Geometry: see drawing. Coordinates: mm, zero at the bounding-box minimum. A direction names the side the tool comes from. Coordinates: 2 decimals unless noted, no trailing zeros. Loops run counter-clockwise (first coordinate to the right, second up) from the corner with the lowest first, then second, coordinate; pieces in that order, holes last. Notation, with made-up numbers: (-19.5, 0.5) -> (3.5, 0.5) arc R22 cw to (3.5, 14.5) -> close; hole circle Ø1 at (-32, 85.5). An arc over 180 degrees is marked (long way). One line per item, written item: value. Start each with the question number.
Item 1: Ray query, probe 1 along Y at (x, z) = (12.7, 4.25); probe 2 along Z at (x, y) = (44.5, 12.7) (3 decimals); probe 3 along Z at (x, y) = (5, 9.5). Return the intervals inside material, ascending. Write a range as from..to.
Item 2: Mould query, pull axis X, two halves, no side actions, for the marked faces 4, 5 and 6. Classes: +X half, -X half, draft (parallel to the pull), parting line (faces both ways), or undercut.
Item 3: Section query D-D on x = 17. Return loops of the section in (y, z).
Item 4: Contact query for flat-ended pins moving along their axis: pin 1 Ø10 at (y, z) = (4.5, 36.5) entering from +X; pin 2 Ø1 at (y, z) = (20, 7.5) entering from -X; pin 3 Ø3 at (y, z) = (7.5, 13) entering from -X; pin 4 Ø11.5 at (y, z) = (12.7, 28.575) entering from -X. Output: stop coordinate, or through.
Item 5: Set-up query: the marked faces 1, 2 and 3. Return all of +Z, -Z, +X, -X, +Y, -Y with unobstructed straight access to the full face (end or side cutting, diameter ignored); none if empty.
Item 6: Section query A-A on y = 17.5. Return loops of the section in (x, z).
Item 7: Section query B-B on z = 32. Return loops of the section in (x, y).
Item 8: Section query C-C on x = 47. Return loops of the section in (y, z) (3 decimals).
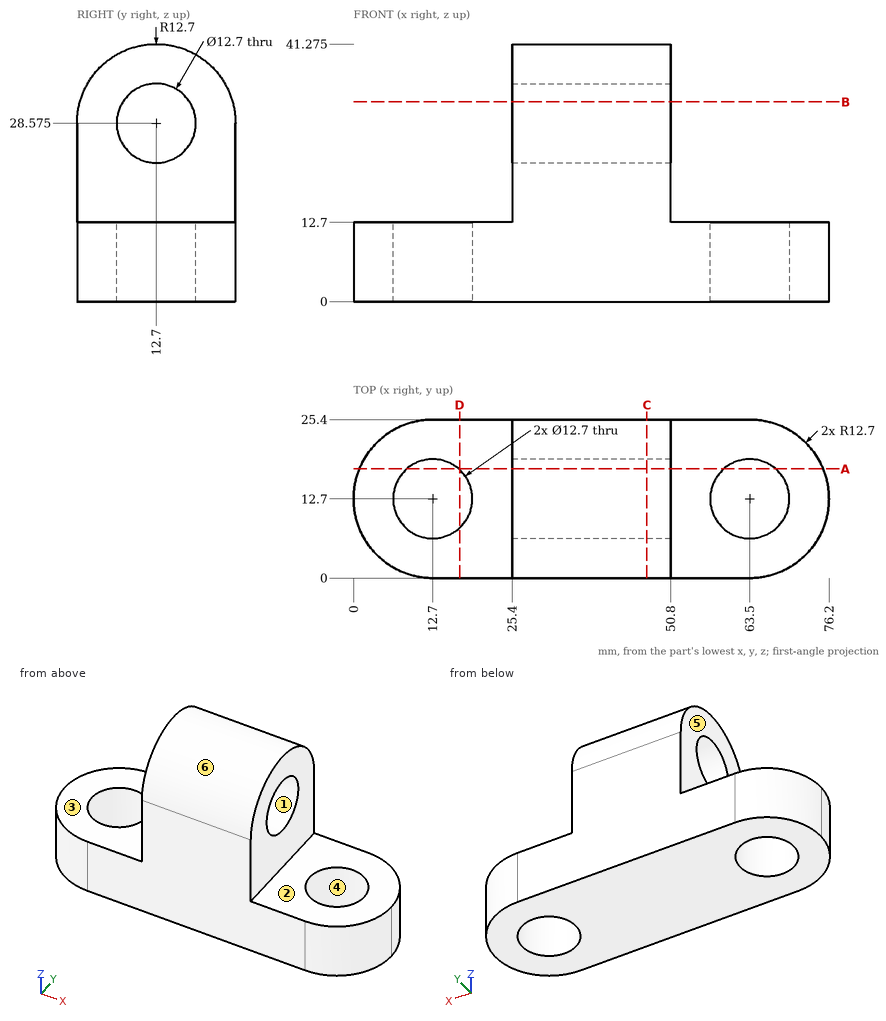
Reply:
1. probe 1: y = 0..6.35, 19.05..25.4
1. probe 2: z = 0..22.225, 34.925..41.275
1. probe 3: z = 0..12.7
2. face 4: undercut
2. face 5: -X half
2. face 6: draft
3. outline: (0, 0) -> (8.03, 0) -> (8.03, 12.7) -> (0, 12.7) -> close; (17.37, 0) -> (25.4, 0) -> (25.4, 12.7) -> (17.37, 12.7) -> close
4. pin 1: stops at x = 50.8
4. pin 2: stops at x = 1.97
4. pin 3: stops at x = 0.56
4. pin 4: passes through
5. face 1: +X, -X
5. face 2: +Z, +X, +Y, -Y
5. face 3: +Z, -X, +Y, -Y
6. outline: (0.94, 0) -> (8.54, 0) -> (8.54, 12.7) -> (0.94, 12.7) -> close; (16.86, 0) -> (59.34, 0) -> (59.34, 12.7) -> (50.8, 12.7) -> (50.8, 24.42) -> (25.4, 24.42) -> (25.4, 12.7) -> (16.86, 12.7) -> close; (25.4, 32.73) -> (50.8, 32.73) -> (50.8, 40.33) -> (25.4, 40.33) -> close; (67.66, 0) -> (75.26, 0) -> (75.26, 12.7) -> (67.66, 12.7) -> close
7. outline: (25.4, 0.47) -> (50.8, 0.47) -> (50.8, 7.35) -> (25.4, 7.35) -> close; (25.4, 18.05) -> (50.8, 18.05) -> (50.8, 24.93) -> (25.4, 24.93) -> close
8. outline: (0, 0) -> (25.4, 0) -> (25.4, 28.575) arc R12.7 ccw to (0, 28.575) -> close; hole circle Ø12.7 at (12.7, 28.575)
